Autodesk Fusion 360 part; units mm, degrees
sketch "Sketch1" plane through (0, 0, 0) normal (0, 0, 1) x (1, 0, 0)
  circle A0 centre (0, 0) radius 21.59 construction
  line L0 (0, 27.546) -> (0, -31.973) construction
  line L1 (-40.4824, 0) -> (36.5438, 0) construction
  line L2 (0, 1.75) -> (0, 22.5)
  line L3 (1.75, 0) -> (22.5, 0)
  line L4 (-2, 1.5) -> (2, 1.5)
  line L5 (-2, -1.5) -> (2, -1.5)
  circle A1 centre (0, 0) radius 5.08
  arc A2 (-2, 1.5) -> (-2, -1.5) centre (0, 0) ccw
  arc A3 (2, -1.5) -> (2, 1.5) centre (0, 0) ccw
  circle A4 centre (0, 13.566) radius 6.5 construction
  circle A5 centre (0, 13.566) radius 2.05
  line L6 (7.62, 20.066) -> (-7.158, 20.066) construction
  line L7 (-11.43, 21.59) -> (19.6746, 21.59) construction
  dimension "d1" = 43.18
  dimension "d3" = 5
  dimension "d4" = 3
  dimension "d5" = 10.16
  dimension "d6" = 2.5
  dimension "d7" = 13
  dimension "d8" = 4.1
  dimension "d18" = 1.524
extrude "Extrude1" add sketch "Sketch1" along normal blind 5.08 makes body 1 at (2.0475, 13.4638, 3.3867) makes body 2 at (5.0737, -0.2532, 3.3867)
pattern_circular "C-Pattern4" count 3 over 360 about axis through (0, 0, 1.75) along (0, 0, 1) of bodies 1 makes body 3 at (-12.6837, -4.9588, 3.3867) makes body 4 at (10.6363, -8.5051, 3.3867)
sketch "Sketch3" plane through (0, 0, 5.08) normal (0, 0, 1) x (-1, 0, 0)
  arc A0 (2, -1.5) -> (2, 1.5) centre (0, 0) ccw
  line L0 (2, -1.5) -> (-2, -1.5)
  arc A1 (-2, 1.5) -> (-2, -1.5) centre (0, 0) ccw
  line L1 (-2, 1.5) -> (2, 1.5)
  circle A2 centre (0, 0) radius 5.08
  line L2 (13.5239, 5.758) -> (1.7754, -14.591)
  line L3 (-1.7754, -14.591) -> (-13.5239, 5.758)
  line L4 (11.7485, 8.833) -> (-11.7485, 8.833)
  circle A3 centre (11.7485, 6.783) radius 2.05
  circle A4 centre (0, -13.566) radius 2.05
  circle A5 centre (-11.7485, 6.783) radius 2.05
extrude "Extrude4" add sketch "Sketch3" along normal blind 2.54 contours A0 L0 A1 L1 | A2 | L2 L3 L4 A3 A4 A5 | A3 | A4 | A5 bodies 1 2 3 4
Check sheet for the modelled part. Datum: model origin and axes. Units: mm. A direction names the side the tool comes from. Give positions to 0.01 mm unless a question says otherwise; leave off trailing zeros. Order: outer loops, then holes, each group sorted by start corner. A loop starts at its lowest first (then second) coordinate and runs counter-clockwise, first axis right, second up. Notation, with made-up numbers: M -16.5,87 L 28.5,87 A17 ccw 28.5,104 Z; hole C 51.25,49 d5. An arc over 180 degrees is marked long. Answer in a Markdown table with one row per item. Add a question column.
Q1. Thickness scan on L1, parallel to Y at x = 1.5, z = 2.75; L2, parallel to Z at x = -0.5, y = 0.75; L3, parallel to X at y = 1.25, z = 2. Record the ranges inside material, lowest first.
Q2. Gauge pin test, flat ends, axial feed: pin 1 Ø1.2 at (x, z) = (0, 3.5) entering from -Y; pin 2 Ø0.9 at (x, y) = (0, -0.5) entering from -Z; pin 3 Ø8 at (x, y) = (-6.5, 6) entering from -Z; pin 4 Ø1.5 at (y, z) = (12.5, 1) entering from +X. Record the tip position at first contact, or that the pin passes through.
Q3. Sectioned sample at D-D, the plane z = 5.75. Record the boundary of the cut face in (x, y).
Q4. Access from +Z, -Z, +X, -X, +Y, -Y to the whole of each face (thin tool, end or side, straight path). Record for faces 1 (the flat face through (0, -2, 0)), 2 (the flat face through (3, -5, 5.08)).
Q5. Sectioned sample at C-C, the plane x = 0. Record the boundary of the cut face in (y, z), and give its area (3 significant figures).
Q6. Sectioned sample at A-A, the plane z = 2.5. Record the boundary of the cut face in (x, y).
Q7. Sectioned sample at B-B, the plane y = -3.5. Record the boundary of the cut face in (x, z), and give its area (3 significant figures).
Q8. Release check for a two-part mould opening along X. For faces 3 (the flat face through (0, 14, 0)), 4 (the flat face through (-7.732, 4.274, 6.332)), 5 (the cylindrical face through (2.5, 0, 2.5)) record: released by +X, released by -X, zero draft, split by the parting line, or undercut.
Verdict:
| question | item | result |
|---|---|---|
| 1 | L1 | -4.85 to -1.5, 1.5 to 4.85, 12.17 to 14.96 |
| 1 | L2 | 5.08 to 7.62 |
| 1 | L3 | -4.92 to -2.17, 2.17 to 4.92 |
| 2 | pin 1 | y = -5.08 |
| 2 | pin 2 | z = 5.08 |
| 2 | pin 3 | z = 0 |
| 2 | pin 4 | x = 2.03 |
| 3 | outline | M -13.52,-5.76 A2.05 ccw -11.75,-8.83 L 11.75,-8.83 A2.05 ccw 13.52,-5.76 L 1.78,14.59 A2.05 ccw -1.78,14.59 Z |
| 4 | face 1 | -Z, +X, -X, +Y, -Y |
| 4 | face 2 | -Z |
| 5 | outline | M -8.83,5.08 L -5.08,5.08 L -5.08,0 L -1.5,0 L -1.5,5.08 L 1.5,5.08 L 1.5,0 L 5.08,0 L 5.08,5.08 L 11.52,5.08 L 11.52,0 L 15.62,0 L 15.62,7.62 L -8.83,7.62 Z |
| 5 | area | 119 mm² |
| 6 | outline | C -11.75,-6.78 d4.1; C 0,0 d10.16; C 0,13.57 d4.1; C 11.75,-6.78 d4.1; hole M -2,-1.5 L 2,-1.5 A2.5 ccw 2,1.5 L -2,1.5 A2.5 ccw Z |
| 7 | outline | M -12.22,5.08 L -3.68,5.08 L -3.68,0 L 3.68,0 L 3.68,5.08 L 12.22,5.08 L 12.22,7.62 L -12.22,7.62 Z |
| 7 | area | 99.5 mm² |
| 8 | face 3 | zero draft |
| 8 | face 4 | released by -X |
| 8 | face 5 | undercut |
